Here's how the part is built. I have some questions about the finished solid (model axes, mm). A direction names the side the tool comes from. Give positions to 0.01 mm unless a question says otherwise; leave off trailing zeros. Loops run counter-clockwise (first coordinate to the right, second up) from the corner with the lowest first, then second, coordinate; pieces in that order, holes last. Notation, with made-up numbers: (61, -18) - (80, -18) arc R18 cw to (80, -13) - close; hole circle Ø9 at (32.5, 24). An arc over 180 degrees is marked (long way). Use one line per item in the form item = value.
from build123d import *

# Parameters (mm, degrees)
SKETCH1_W           = 30
SKETCH1_H           = 30
BOSS_EXTRUDE1_DEPTH = 30
SKETCH2_R           = 10
BOSS_EXTRUDE2_DEPTH = 400
SKETCH3_W           = 30
SKETCH3_H           = 30
BOSS_EXTRUDE3_DEPTH = 30
SKETCH4_R           = 10
CUT_EXTRUDE1_DEPTH  = 30


with BuildPart() as part:
    # Sketch1 → Boss-Extrude1 (new body)
    with BuildSketch(Plane(origin=(0, 0, 0), x_dir=(0, 0, -1), z_dir=(1, 0, 0))):
        Rectangle(SKETCH1_W, SKETCH1_H)
    extrude(amount=BOSS_EXTRUDE1_DEPTH)

    # Sketch2 → Boss-Extrude2 (add)
    with BuildSketch(Plane(origin=(30, 0, 0), x_dir=(0, 0, -1), z_dir=(1, 0, 0))):
        Circle(SKETCH2_R)
    extrude(amount=BOSS_EXTRUDE2_DEPTH)

    # Sketch3 → Boss-Extrude3 (add)
    with BuildSketch(Plane(origin=(430, 0, 0), x_dir=(0, 0, -1), z_dir=(1, 0, 0))):
        Rectangle(SKETCH3_W, SKETCH3_H)
    extrude(amount=BOSS_EXTRUDE3_DEPTH)

    # Sketch4 → Cut-Extrude1 (cut)
    with BuildSketch(Plane(origin=(0, 15, 0), x_dir=(1, 0, 0), z_dir=(0, 1, 0))):
        with Locations((445, 0)):
            Circle(SKETCH4_R)
    extrude(amount=-CUT_EXTRUDE1_DEPTH, mode=Mode.SUBTRACT)


solid = part.part
(1) Thinking about a two-plate mould opening in X: for faces 3 (the flat face through (430, 10.2, 0.2)), 4 (the flat face through (445, 0, -15)), 5 (the flat face through (460, 0, 0)), which applies, pulls with the +X half, pulls with the -X half, needs draft (parallel to the pull), parting line crosses it, or undercut?
Geometry says:
face_3 = undercut
face_4 = needs draft
face_5 = pulls with the +X half
(2) For P1, Ø5, axis at x = 309.5, y = -5, coming from the +Z side; P2, Ø12, axis at x = 125, z = -2.5, coming from the -Y side; P3, Ø6, axis at x = 277, y = 0.5, coming from the -Z side, each with a flat end and sliding along its axis, tell me the tip position at first contact or that it passes through.
Geometry says:
P1 = 9.68
P2 = -10
P3 = -10
(3) If we section it at D-D (x = 312.5): List the corners of the cut face in (y, z) for me, plus the area to 3 significant figures.
Geometry says:
outline = circle Ø20 at (0, 0)
area = 314 mm²
(4) If we section it at C-C (y = 6): List the corners of the cut face in (x, z) for me.
Geometry says:
outline = (0, -15) - (30, -15) - (30, -8) - (430, -8) - (430, -15) - (460, -15) - (460, 15) - (430, 15) - (430, 8) - (30, 8) - (30, 15) - (0, 15) - close; hole circle Ø20 at (445, 0)
(5) If we section it at B-B (z = 0): List the corners of the cut face in (x, y) for me, plus the area to 3 significant figures.
Geometry says:
outline = (0, -15) - (30, -15) - (30, -10) - (430, -10) - (430, -15) - (435, -15) - (435, 15) - (430, 15) - (430, 10) - (30, 10) - (30, 15) - (0, 15) - close; (455, -15) - (460, -15) - (460, 15) - (455, 15) - close
area = 9,200 mm²
(6) For faces 1 (the cylindrical face through (227.2, -9.76, 2.17)), 2 (the flat face through (0, 0, 0)), which set-ups out of +Z, -Z, +X, -X, +Y, -Y let a thin tool reach every point of the face, with its end or its side?
Geometry says:
face_1 = none
face_2 = +Z, -Z, -X, +Y, -Y
(7) If I drill on probe 1 along X at (y, z) = (-10.5, 0.25); probe 2 along X at (y, z) = (-13.25, 11.25); probe 3 along Z at (x, y) = (445, 3.5), over which ranges is the centre line in solid material (lowest first)?
Geometry says:
probe_1 = 0 to 30, 430 to 435, 455 to 460
probe_2 = 0 to 30, 430 to 460
probe_3 = -15 to -10, 10 to 15
(8) If we section it at A-A (x = 445): List the corners of the cut face in (y, z) for me.
Geometry says:
outline = (-15, -15) - (15, -15) - (15, -10) - (-15, -10) - close; (-15, 10) - (15, 10) - (15, 15) - (-15, 15) - close
